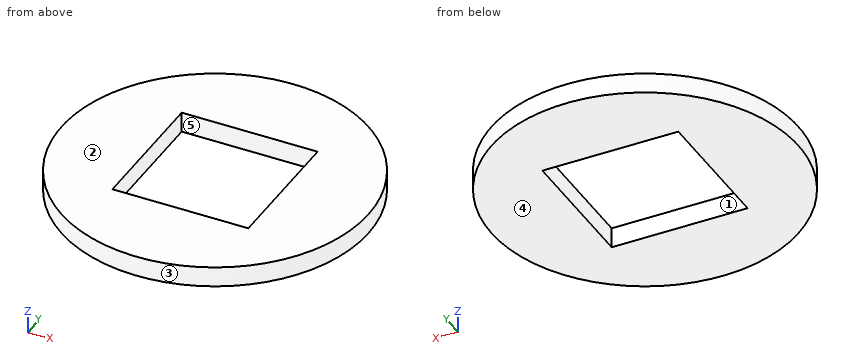
```python
from build123d import *

# Parameters (mm, degrees)
SKETCH1_R           = 7.5
SKETCH1_W           = 6.65
SKETCH1_H           = 6.65
BOSS_EXTRUDE1_DEPTH = 0.5


with BuildPart() as part:
    # Sketch1 → Boss-Extrude1 (new, symmetric)
    with BuildSketch(Plane.XY):
        Circle(SKETCH1_R)
        Rectangle(SKETCH1_W, SKETCH1_H, mode=Mode.SUBTRACT)
    extrude(amount=BOSS_EXTRUDE1_DEPTH, both=True)


solid = part.part
```
Model file for the job. Use its own axes, mm. Face numbers are marked on the shaded views. A direction names the side the tool comes from. Give positions to 0.01 mm unless a question says otherwise; leave off trailing zeros. Loops run counter-clockwise (first coordinate to the right, second up) from the corner with the lowest first, then second, coordinate; pieces in that order, holes last. Notation, with made-up numbers: (38, 21) - (72, 21) arc R17 cw to (72, 39) - close; hole circle Ø6 at (66, -28). An arc over 180 degrees is marked (long way). One line per item, written item: value. Start each with the question number.
1. Pin check, flat tips, straight feed: pin 1 (0.5 mm diameter, centred on y = -0.5, z = 0, fed in from -X); pin 2 (0.5 mm diameter, centred on x = -0.5, z = 0, fed in from -Y). Stop position of each tip, or through.
2. Slice it at D-D (x = 4.5). List the corners of the cut face in (y, z).
3. Slice it at A-A (y = 0). List the corners of the cut face in (x, z) (3 decimals).
4. Slice it at C-C (z = -0.2). List the corners of the cut face in (x, y) (3 decimals).
5. Probe L1, parallel to Y at x = 0, z = 0.35 (3 decimals); L2, parallel to X at y = 2.75, z = 0.45 (3 decimals); L3, parallel to X at y = -2.5, z = 0.15 (3 decimals). List the from-to ranges inside material, lowest first. Write a range as from..to.
6. Pull direction X, two halves, no side cores. Call the marked faces 3, 4 and 5: pulls with the +X half, pulls with the -X half, needs draft (parallel to the pull), parting line crosses it, or undercut.
7. Which spindle directions (+Z, -Z, +X, -X, +Y, -Y) get a long thin tool onto all of the face, cutting with end or side? Do the marked faces 1 and 2. Say none if no direction does.
Solution:
1. pin 1: stops at x = -7.5
1. pin 2: stops at y = -7.5
2. outline: (-6, -0.5) - (6, -0.5) - (6, 0.5) - (-6, 0.5) - close
3. outline: (-7.5, -0.5) - (-3.325, -0.5) - (-3.325, 0.5) - (-7.5, 0.5) - close; (3.325, -0.5) - (7.5, -0.5) - (7.5, 0.5) - (3.325, 0.5) - close
4. outline: circle Ø15 at (0, 0); hole (-3.325, -3.325) - (3.325, -3.325) - (3.325, 3.325) - (-3.325, 3.325) - close
5. L1: y = -7.5..-3.325, 3.325..7.5
5. L2: x = -6.978..-3.325, 3.325..6.978
5. L3: x = -7.071..-3.325, 3.325..7.071
6. face 3: parting line crosses it
6. face 4: needs draft
6. face 5: undercut
7. face 1: +Z, -Z
7. face 2: +Z, +X, -X, +Y, -Y
